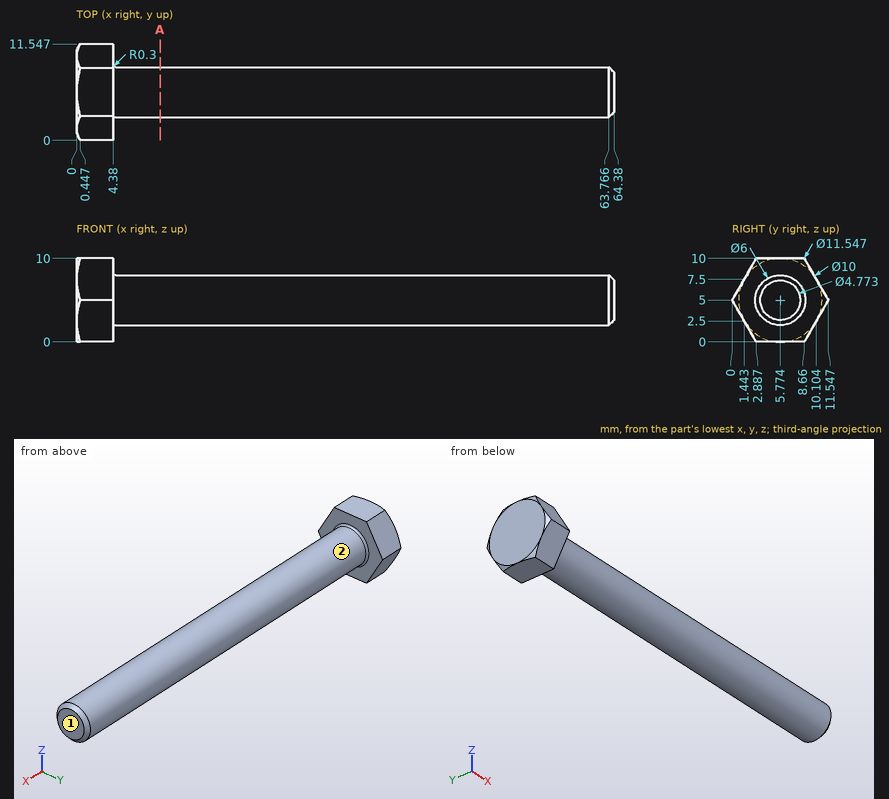
The drawing under review shows one solid part. Ordinate dimensions are in mm from its lowest x, y, z. A direction names the side the tool comes from. Round coordinates to 2 decimals unless told otherwise and drop trailing zeros. Loops run counter-clockwise (first coordinate to the right, second up) from the corner with the lowest first, then second, coordinate; pieces in that order, holes last. Notation, with made-up numbers: (29.5, 86) -> (69.5, 86) arc R23 cw to (69.5, 112) -> close; hole circle Ø10 at (23, 81.25). An arc over 180 degrees is marked (long way). Answer in a Markdown table with one row per item.
1) Consider section A-A, the plane x = 10. Write out the cut boundary in (y, z).
Taken from the geometry:
| item | result |
|---|---|
| outline | circle Ø6 at (5.77, 5) |
2) Tool access review of the marked faces 1 and 2: name each direction out of +Z, -Z, +X, -X, +Y, -Y from which nothing blocks a thin tool from reaching the whole face with its end or side.
Taken from the geometry:
| item | result |
|---|---|
| face 1 | +Z, -Z, +X, +Y, -Y |
| face 2 | +X |
3) Wall thickness on line 1 along X through (y, z) = (6, 9.25); line 2 along X through (y, z) = (3.5, 4.25) (1 decimal); line 3 along Z through (x, y) = (13, 6): over which ranges is each line inside the solid? List them lowest first.
Taken from the geometry:
| item | result |
|---|---|
| line 1 | x = 0 to 4.38 |
| line 2 | x = 0 to 64.4 |
| line 3 | z = 2.01 to 7.99 |
4) For pin 1 Ø3 at (x, z) = (32, 9) entering from +Y; pin 2 Ø1.5 at (x, z) = (42, 7.5) entering from +Y; pin 3 Ø4 at (x, z) = (13, 6) entering from +Y, all flat-tipped, find the tip position at first contact; note any pin that passes through.
Taken from the geometry:
| item | result |
|---|---|
| pin 1 | stops at y = 7.43 |
| pin 2 | stops at y = 8.21 |
| pin 3 | stops at y = 8.77 |
